For this review, take the finished solid that the model builds, in its own axes (mm). A direction names the side the tool comes from. Give positions to 0.01 mm unless a question says otherwise; leave off trailing zeros. Order: outer loops, then holes, each group sorted by start corner. A loop starts at its lowest first (then second) coordinate and runs counter-clockwise, first axis right, second up. Notation, with made-up numbers: M 36.5,81.5 L 49.5,81.5 A21 cw 49.5,85.5 Z; hole C 69.25,-6.5 d10. An arc over 180 degrees is marked long. Use CSV: the item, a comma, the result in double quotes. Start each with the question number.
(1) Consider section C-C (y = 25.5). Write out the cut boundary in (x, z), and give its area (3 significant figures).
(2) Tool access review of faces 1 (the face through (-6.528, 0.515, 31.254)), 2 (the face through (31, 19, 20.504)), 3 (the face through (6, 37.58, 27.18)), 4 (the face through (-10.295, 15, 1)), 5 (the face through (6.256, 18.798, 26.35)): name each direction out of +Z, -Z, +X, -X, +Y, -Y from which nothing blocks a thin tool from reaching the whole face with its end or side.
(3) Draft analysis for pull direction X (two halves, no side actions). For faces 6 (the face through (6, 0.52, 27.18)), 7 (the face through (-7.927, 0.515, 33.005)), 8 (the face through (-6.528, 37.585, 31.254)), 9 (the face through (5.89, 0.515, 29.661)), state which applies: pulls with the +X half, pulls with the -X half, needs draft (parallel to the pull), parting line crosses it, or undercut.
(4) Consider section D-D (z = 5). Write out the cut boundary in (x, y).
(5) Consider section A-A (y = 19.05). Write out the cut boundary in (x, z), and give its area (3 significant figures).
(6) Wall thickness on L1, parallel to X at y = 11, z = 17; L2, parallel to Z at x = 27, y = 13; L3, parallel to X at y = 3.5, z = 18.5: over which ranges is each line inside the solid? List them lowest first. Write a range as from..to.
(7) Consider section B-B (z = 22). Write out the cut boundary in (x, y).
(8) Clearance check with flat-ended pins moving along their axes: P1, Ø5.5, axis at y = 19.05, z = -4.83, coming from the +X side; P2, Ø7.5, axis at x = 34, y = 20, coming from the +Z side; P3, Ø13.5, axis at x = 24.5, y = 23.5, coming from the -Z side. State where each tip first meets the part, or that it passes through.
Autodesk Inventor part; units mm, degrees
ref_plane "YZ Plane" through (0, 0, 0) normal (1, 0, 0) x (0, 1, 0)
ref_plane "XZ Plane" through (0, 0, 0) normal (0, 1, 0) x (-1, 0, 0)
ref_plane "XY Plane" through (0, 0, 0) normal (0, 0, 1) x (1, 0, 0)
sketch "Sketch1" plane through (0, 0, 0) normal (0, 1, 0) x (-1, 0, 0)
  line L0 (10.2949, -23.8768) -> (10.2949, 26.9232)
  line L1 (10.2949, 26.9232) -> (6.4648, 39.5536)
  line L2 (6.4648, 39.5536) -> (-18.9352, 20.5036)
  line L3 (-18.9352, 20.5036) -> (-44.3352, 20.5036)
  line L4 (-44.3352, 20.5036) -> (-44.3352, 17.9636)
  line L5 (-44.3352, 17.9636) -> (-17.0011, 17.9636)
  line L6 (-17.0011, 17.9636) -> (4.7948, 34.9742)
  line L7 (4.7948, 34.9742) -> (7.7549, 25.8478)
  line L8 (7.7549, 25.8478) -> (7.7549, -23.8768)
  line L9 (7.7549, -23.8768) -> (10.2949, -23.8768)
  point P0 (0, 0)
  dimension "d0" = 19.05
  dimension "d1" = 25.4
  dimension "d2" = 50.8
  dimension "d3" = 70
  dimension "d4" = 70
  dimension "d5" = 2.54
  dimension "d6" = 2.54
  dimension "d7" = 25.4
extrude "Extrusion1" add sketch "Sketch1" along normal blind 38.1
sketch "Sketch2" plane through (-10.2949, 0, -23.8768) normal (-1, 0, 0) x (0, 0, 1)
  line L0 (19.05, 19.05) -> (25.4, 19.05) construction
  line L1 (25.4, 19.05) -> (25.4, 0) construction
  line L2 (0, 0) -> (50.8, 0) construction
  line L3 (19.05, 19.05) -> (0, 19.05) construction
  line L4 (0, 0) -> (0, 38.1) construction
  point P0 (23.8768, 0)
  dimension "d10" = 19.05
  dimension "d11" = 6.35
  dimension "d12" = 19.05
hole "Hole1" at (-10.2949, 19.05, -4.8268) at (-10.2949, 19.05, 1.5232) direction (1, 0, 0) diameter 4.9784 end through all
chamfer "Chamfer1" distance 1.016 angle 45 20 edges at (-10.2949, 0, 1.5232) (-8.3798, 0, 33.2384) (6.2352, 0, 30.0286) (31.6352, 0, 20.5036) (44.3352, 0, 19.2336) (30.6682, 0, 17.9636) (6.1031, 0, 26.4689) (-6.2749, 0, 30.411) (-7.7549, 0, 0.9855) (-9.0249, 0, -23.8768) (31.6352, 38.1, 20.5036) (44.3352, 38.1, 19.2336) (30.6682, 38.1, 17.9636) (6.2352, 38.1, 30.0286) (6.1031, 38.1, 26.4689) (-6.2749, 38.1, 30.411) (-8.3798, 38.1, 33.2384) (-7.7549, 38.1, 0.9855) (-10.2949, 38.1, 1.5232) (-9.0249, 38.1, -23.8768)
properties part number "Encoder Mount"
Check result:
1,outline,"M -10.29,-23.88 L -7.75,-23.88 L -7.75,25.85 L -4.79,34.97 L 17,17.96 L 44.34,17.96 L 44.34,20.5 L 18.94,20.5 L -6.46,39.55 L -10.29,26.92 Z"
1,area,"314 mm^2"
2,face 1,"-Z, -Y"
2,face 2,"+Z, +X, +Y, -Y"
2,face 3,"-Z, +Y"
2,face 4,"+Z, -Z, -X, +Y, -Y"
2,face 5,"-Z, +Y, -Y"
3,face 6,"undercut"
3,face 7,"pulls with the -X half"
3,face 8,"undercut"
3,face 9,"pulls with the +X half"
4,outline,"M -10.29,1.02 L -9.28,0 L -8.77,0 L -7.75,1.02 L -7.75,37.08 L -8.77,38.1 L -9.28,38.1 L -10.29,37.08 Z"
5,outline,"M -10.29,-23.88 L -7.75,-23.88 L -7.75,-7.32 L -10.29,-7.32 Z; M -10.29,-2.34 L -7.75,-2.34 L -7.75,-0.97 L -10.29,-0.97 Z; M -10.29,4.01 L -7.75,4.01 L -7.75,25.85 L -4.79,34.97 L 17,17.96 L 44.34,17.96 L 44.34,20.5 L 18.94,20.5 L -6.46,39.55 L -10.29,26.92 Z"
5,area,"288 mm^2"
6,L1,"x = -10.29..-7.75"
6,L2,"z = 17.96..20.5"
6,L3,"x = -10.29..-7.75, 16.31..44.34"
7,outline,"M -10.29,1.02 L -9.28,0 L -8.77,0 L -7.75,1.02 L -7.75,37.08 L -8.77,38.1 L -9.28,38.1 L -10.29,37.08 Z; M 11.83,1.02 L 13.48,0 L 15.25,0 L 16.94,1.02 L 16.94,37.08 L 15.25,38.1 L 13.48,38.1 L 11.83,37.08 Z"
8,P1,"stops at x = -7.75"
8,P2,"stops at z = 20.5"
8,P3,"stops at z = 17.96"
